The figure shows three views and two pictorial views of one solid part (mm, origin at its lowest corner). Answer the questions. Give positions to 0.01 mm unless a question says otherwise; leave off trailing zeros. Loops run counter-clockwise (first coordinate to the right, second up) from the corner with the lowest first, then second, coordinate; pieces in that order, holes last. Notation, with made-up numbers: (84, 27) -> (108, 27) arc R11 cw to (108, 31) -> close; hole circle Ø4 at (0.5, 18.5). An arc over 180 degrees is marked (long way). Answer as CSV lines item,"result". Start each with the question number.
1. Find section B-B, the plane x = 2.75. Give the vertices of the cut face in (y, z), and give its area (3 significant figures).
2. Find section D-D, the plane x = 12. Give the vertices of the cut face in (y, z), and give its area (3 significant figures).
3. Find section A-A, the plane x = 17. Give the vertices of the cut face in (y, z), and give its area (3 significant figures).
4. Find the intervals of material crossed by line 1 along Y through (x, z) = (4.75, 1.05); line 2 along Y through (x, z) = (13.5, 3); line 3 along Y through (x, z) = (11.5, 1.5), in increasing order.
5. Flat-ended cylindrical pins translate along their axes: pin 1 Ø8 at (x, y) = (10, 67) entering from +Z; pin 2 Ø2 at (y, z) = (24, 2.5) entering from +X; pin 3 Ø10 at (x, y) = (17, 23) entering from -Z; pin 4 Ø1.1 at (y, z) = (48, 1.5) entering from -X. Find the tip coordinate at first contact, or state that the pin passes through.
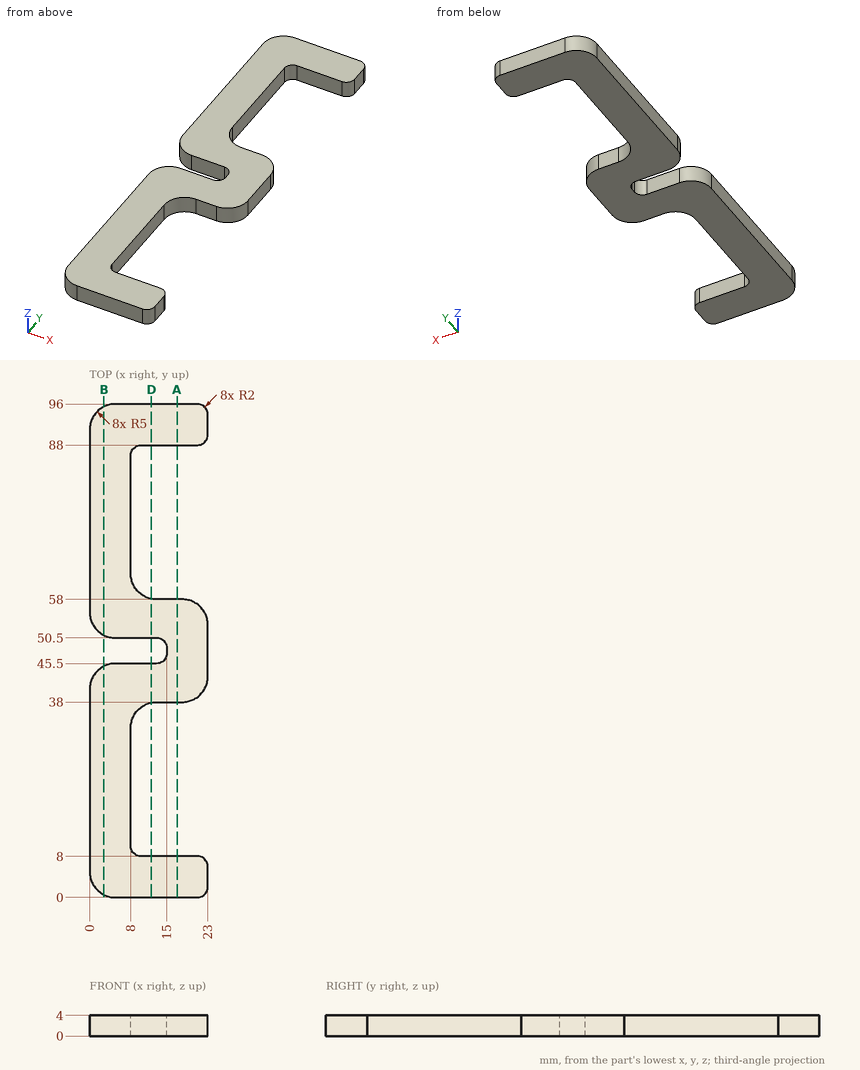
Resolved:
1,outline,"(0.53, 0) -> (44.97, 0) -> (44.97, 4) -> (0.53, 4) -> close; (51.03, 0) -> (95.47, 0) -> (95.47, 4) -> (51.03, 4) -> close"
1,area,"355 mm^2"
2,outline,"(0, 0) -> (8, 0) -> (8, 4) -> (0, 4) -> close; (37.9, 0) -> (45.5, 0) -> (45.5, 4) -> (37.9, 4) -> close; (50.5, 0) -> (58.1, 0) -> (58.1, 4) -> (50.5, 4) -> close; (88, 0) -> (96, 0) -> (96, 4) -> (88, 4) -> close"
2,area,"125 mm^2"
3,outline,"(0, 0) -> (8, 0) -> (8, 4) -> (0, 4) -> close; (38, 0) -> (58, 0) -> (58, 4) -> (38, 4) -> close; (88, 0) -> (96, 0) -> (96, 4) -> (88, 4) -> close"
3,area,"144 mm^2"
4,line 1,"y = 0.01 to 45.49, 50.51 to 95.99"
4,line 2,"y = 0 to 8, 38 to 45.56, 50.44 to 58, 88 to 96"
4,line 3,"y = 0 to 8, 37.77 to 45.5, 50.5 to 58.23, 88 to 96"
5,pin 1,"stops at z = 4"
5,pin 2,"stops at x = 8"
5,pin 3,"passes through"
5,pin 4,"stops at x = 15"
